CAD build for the part. Positions are in the model's coordinates, mm. A direction names the side the tool comes from. Coordinates: 2 decimals unless noted, no trailing zeros. Write each loop counter-clockwise with the first axis right and the second up, starting at its lowest first coordinate (ties: lowest second). Pieces come first, ordered by that corner, then holes. Notation, with made-up numbers: (24.25, 74) -> (49.25, 74) arc R22 ccw to (49.25, 82) -> close; hole circle Ø9 at (53, 12). An arc over 180 degrees is marked (long way). Answer as CSV lines item,"result". Start each with the question number.
```python
from build123d import *

# Parameters (mm, degrees)
F1_DEPTH  = 25
F2_DEPTH  = 5
F3_R      = 5
F5_DEPTH  = 5
F6_W      = 25
F6_H      = 37.5846914337
F10_R     = 1.55
F11_DEPTH = 10
F14_DEPTH = 1
F15_DEPTH = 1
F16_DEPTH = 5
F17_DEPTH = 5


# Not quite as in the source:
# - a feature names something its author has since deleted; it is built from what else it names


with BuildPart() as f1:
    # F0 (on Right) → F1 (new body)
    with BuildSketch(Plane.YZ):
        Polygon((-1.9545168432, 38.6489601963), (-33.5964987424, 14.1788767986), (-28.2257758369, -25.4589250511), (-8.406874912, -22.7735635983), (-0.7535947717, -79.2574312341), (4.2011304595, -78.5860908709), (0.1149024355, -48.4283077234), (-0.6409071668, -42.8501701471), (-3.9713255886, -18.2705245759), (3.1545996335, -0.8816359607), (10.2805248557, 16.5072526545), (30.8972257421, 32.4510197574), (34.3548171712, 35.1249215027), (58.4291094867, 53.742590351), (55.370349062, 57.6978380884), (10.2805248557, 22.8279692467), align=None)
        Polygon((-25.8654488138, -5.6400241263), (-7.3142972833, -13.2422419285), (-9.1963342424, -17.8348428934), (-23.9423909688, -19.8328594567), align=None, mode=Mode.SUBTRACT)
        Polygon((1.5615552233, 8.4168698067), (-1.4719884671, 1.0143288458), (-4.5055321574, -6.3882121151), (-5.26391808, -8.2388473554), (-11.7411414209, -5.5844966263), (-17.2930471416, -3.3093388585), (-23.7702704824, -0.6549881294), (-23.0118845598, 1.1956471108), (-16.944797179, 16.0007290327), (-16.1864112564, 17.851364273), (-9.7091879156, 15.1970135439), (-4.1572821949, 12.9218557761), (2.3199411459, 10.267505047), align=None, mode=Mode.SUBTRACT)
        Polygon((-14.6534166938, 22.50764705), (-2.8510041559, 31.6349520341), (6.2523573083, 19.863500585), (4.1741345282, 14.7921613112), align=None, mode=Mode.SUBTRACT)
        Polygon((-10.4675738382, 13.3463783036), (-4.9156681175, 11.0712205358), (-4.1572821949, 12.9218557761), (-9.7091879156, 15.1970135439), align=None)
        Polygon((-11.7411414209, -5.5844966263), (-10.9827554983, -3.7338613861), (-16.534661219, -1.4587036183), (-17.2930471416, -3.3093388585), align=None)
        Polygon((43.3848339814, 23.4483111776), (34.3548171712, 35.1249215027), (30.8972257421, 32.4510197574), (37.9390681356, 23.3452947817), (11.4856577492, -41.2070815569), (-0.6409071668, -42.8501701471), (0.1149024355, -48.4283077234), (14.7421520123, -46.4463889317), align=None)
    extrude(amount=F1_DEPTH)

    # F0 (on Right) → F2 (join)
    with BuildSketch(Plane.YZ):
        Polygon((-16.944797179, 16.0007290327), (-10.4675738382, 13.3463783036), (-9.7091879156, 15.1970135439), (-16.1864112564, 17.851364273), align=None)
        Polygon((-4.9156681175, 11.0712205358), (1.5615552233, 8.4168698067), (2.3199411459, 10.267505047), (-4.1572821949, 12.9218557761), align=None)
        Polygon((-17.2930471416, -3.3093388585), (-16.534661219, -1.4587036183), (-23.0118845598, 1.1956471108), (-23.7702704824, -0.6549881294), align=None)
        Polygon((-5.26391808, -8.2388473554), (-4.5055321574, -6.3882121151), (-10.9827554983, -3.7338613861), (-11.7411414209, -5.5844966263), align=None)
    extrude(amount=F2_DEPTH)

    # F3
    f3_edges = [f1.edges().sort_by_distance(p)[0] for p in [
        (12.5, -33.596499, 14.178877),
    ]]
    fillet(f3_edges, radius=F3_R)

    # F4 (on face) → F5 (cut)
    with BuildSketch(Plane(origin=(0, 28.9192447, -11.8510377387), x_dir=(-1, 0, 0), z_dir=(0, 0.9253176201, -0.3791929613))):
        Polygon((-25, 33.3185826418), (-25, -32.5577652662), (-18.2082508509, 0.3804086878), align=None)
        Polygon((-14.2606471901, -5.2335595779), (-20, -32.3875417919), (-4.8253758508, -32.3875417919), align=None)
        Polygon((-11.0385, 0.3804086878), (0, -31.3875417919), (0, 32.1483591675), align=None)
        with BuildLine():
            ThreePointArc((-13.1233754255, 0.3804086878), (-14.6233754255, 1.8804086878), (-16.1233754255, 0.3804086878))
            Line((-16.1233754255, 0.3804086878), (-13.1233754255, 0.3804086878))
        make_face()
        with BuildLine():
            Line((-13.1233754255, 0.3804086878), (-16.1233754255, 0.3804086878))
            ThreePointArc((-16.1233754255, 0.3804086878), (-14.6233754255, -1.1195913122), (-13.1233754255, 0.3804086878))
        make_face()
        Polygon((-5, 33.1483591675), (-20, 33.1483591675), (-14.3256804669, 6.3097710203), align=None)
    extrude(amount=-F5_DEPTH, mode=Mode.SUBTRACT)

    # F8 (on offset) → F9 section 0
    with BuildSketch(Plane(origin=(0, 12.2635275379, -5.0255644353), x_dir=(-1, 0, 0), z_dir=(0, 0.9253176201, -0.3791929613))):
        with BuildLine():
            ThreePointArc((-17.1248646707, 2.8558931882), (-18.1499909365, 0.381019454), (-17.1248646707, -2.0938542801))
            ThreePointArc((-17.1248646707, -2.0938542801), (-14.6499909365, -3.118980546), (-12.1751172024, -2.0938542801))
            ThreePointArc((-12.1751172024, -2.0938542801), (-11.1499909365, 0.381019454), (-12.1751172024, 2.8558931882))
            ThreePointArc((-12.1751172024, 2.8558931882), (-14.6499909365, 3.881019454), (-17.1248646707, 2.8558931882))
        make_face()
    # F6 (on face) → F9 section 1
    with BuildSketch(Plane(origin=(0, 3.0103513367, -1.2336348224), x_dir=(-1, 0, 0), z_dir=(0, 0.9253176201, -0.3791929613))):
        with Locations((-12.5, 0.3804086878)):
            Rectangle(F6_W, F6_H)
    loft()

    # F10 (on face) → F11 (cut)
    with BuildSketch(Plane(origin=(0, 12.2635275379, -5.0255644353), x_dir=(-1, 0, 0), z_dir=(0, 0.9253176201, -0.3791929613))):
        with Locations((-14.6499909461, 0.3810196067)):
            Circle(F10_R)
    extrude(amount=-F11_DEPTH, mode=Mode.SUBTRACT)

    # F13 (on face) → F14 (join)
    with BuildSketch(Plane(origin=(0, -11.2853910764, -1.5291137632), x_dir=(1, 0, 0), z_dir=(0, -0.9909450462, -0.1342680726))):
        with BuildLine():
            ThreePointArc((14, -43.6885751417), (16, -45.6885751417), (18, -43.6885751417))
            ThreePointArc((18, -43.6885751417), (16, -41.6885751417), (14, -43.6885751417))
        make_face()
        with BuildLine():
            Line((18, -56.1885751417), (18, -43.6885751417))
            ThreePointArc((18, -43.6885751417), (16, -45.6885751417), (14, -43.6885751417))
            Line((14, -43.6885751417), (14, -56.1885751417))
            ThreePointArc((14, -56.1885751417), (16, -54.1885751417), (18, -56.1885751417))
        make_face()
        with BuildLine():
            ThreePointArc((14, -56.1885751417), (16, -58.1885751417), (18, -56.1885751417))
            ThreePointArc((18, -56.1885751417), (16, -54.1885751417), (14, -56.1885751417))
        make_face()
    extrude(amount=F14_DEPTH)

    # F12 (on face) → F15 (join)
    with BuildSketch(Plane(origin=(0, -7.1996627103, 9.3098006026), x_dir=(1, 0, 0), z_dir=(0, -0.6117520849, 0.7910495475))):
        with BuildLine():
            ThreePointArc((14, 56.8474623166), (16, 54.8474623166), (18, 56.8474623166))
            ThreePointArc((18, 56.8474623166), (16, 58.8474623166), (14, 56.8474623166))
        make_face()
        with BuildLine():
            Line((18, 44.3474623166), (18, 56.8474623166))
            ThreePointArc((18, 56.8474623166), (16, 54.8474623166), (14, 56.8474623166))
            Line((14, 56.8474623166), (14, 44.3474623166))
            ThreePointArc((14, 44.3474623166), (16, 46.3474623166), (18, 44.3474623166))
        make_face()
        with BuildLine():
            ThreePointArc((14, 44.3474623166), (16, 42.3474623166), (18, 44.3474623166))
            ThreePointArc((18, 44.3474623166), (16, 46.3474623166), (14, 44.3474623166))
        make_face()
    extrude(amount=F15_DEPTH)

    # F12 (on face) → F16 (cut)
    with BuildSketch(Plane(origin=(0, -7.1996627103, 9.3098006026), x_dir=(1, 0, 0), z_dir=(0, -0.6117520849, 0.7910495475))):
        with BuildLine():
            ThreePointArc((14, 64.8474623166), (16, 62.8474623166), (18, 64.8474623166))
            ThreePointArc((18, 64.8474623166), (16, 66.8474623166), (14, 64.8474623166))
        make_face()
        with BuildLine():
            ThreePointArc((14, 36.3474623166), (16, 34.3474623166), (18, 36.3474623166))
            ThreePointArc((18, 36.3474623166), (16, 38.3474623166), (14, 36.3474623166))
        make_face()
    extrude(amount=-F16_DEPTH, mode=Mode.SUBTRACT)

    # F13 (on face) → F17 (cut)
    with BuildSketch(Plane(origin=(0, -11.2853910764, -1.5291137632), x_dir=(1, 0, 0), z_dir=(0, -0.9909450462, -0.1342680726))):
        with BuildLine():
            ThreePointArc((14, -35.6885751417), (16, -37.6885751417), (18, -35.6885751417))
            ThreePointArc((18, -35.6885751417), (16, -33.6885751417), (14, -35.6885751417))
        make_face()
        with BuildLine():
            ThreePointArc((14, -64.1885751417), (16, -66.1885751417), (18, -64.1885751417))
            ThreePointArc((18, -64.1885751417), (16, -62.1885751417), (14, -64.1885751417))
        make_face()
    extrude(amount=-F17_DEPTH, mode=Mode.SUBTRACT)


solid = f1.part
```
1. Wall check: line 1 (Y direction, x = 13, z = 24); line 2 (Y direction, x = 12.5, z = -14.5); line 3 (Z direction, x = 8.5, y = 0). Give the ranges that are in metal, low to high.
2. Cut at C-C (z = 40). Give the cut face in (x, y).
3. Cut at A-A (z = -27.5). Give the cut face in (x, y).
4. Tool access for faces 4 (the face through (12.32, 7.33, -47.45)), 5 (the face through (5, -13, 16)), 6 (the face through (12.325, -5.108, 18.596)), 7 (the face through (14.672, 3.163, -0.861)), 8 (the face through (15.972, 32.305, 41.125)): list every direction of +Z, -Z, +X, -X, +Y, -Y with a clear straight run to the whole face (end or side of a thin tool).
5. Flat gauge pins, fed straight in: P1, Ø1, axis at x = 22, z = 41, coming from the +Y side; P2, Ø4, axis at x = 22, y = 35.5, coming from the -Z side; P3, Ø1.4, axis at y = -2.5, z = 11, coming from the +X side. Where does each tip first touch, or does it go through?
6. Mould opens along X. For faces 1 (the face through (12.32, 1.64, 25.83)), 2 (the face through (14, -5, -51)), 3 (the face through (14, -4.1, -36.5)) say: pulls with the +X half, pulls with the -X half, needs draft (parallel to the pull), parting line crosses it, or undercut.
7. Cut at B-B (x = 8.75). Count the separate pieces of the cut face and the enclosed holes in it, then the cut area to 3 significant figures.
Geometry check:
1,line 1,"-20.9 to -12.72, 3.05 to 9.37, 11.8 to 19.97, 37.43 to 42.96"
1,line 2,"-29.71 to -24.66, -7.83 to 1.5, 22.43 to 27.83"
1,line 3,"-79.16 to -42.76, -15.5 to 4.61, 11.22 to 16.5, 27.95 to 36.12"
2,outline,"(0, 32.49) -> (14, 32.49) -> (14, 30.85) -> (18, 30.85) -> (18, 32.49) -> (25, 32.49) -> (25, 40.66) -> (0, 40.66) -> close"
3,outline,"(0, -7.77) -> (25, -7.77) -> (25, -2.72) -> (0, -2.72) -> close; (4.32, 17.1) -> (9.49, 17.1) -> (10.2, 22.51) -> (5.03, 22.51) -> close; (16.73, 22.51) -> (17.16, 17.1) -> (22.2, 17.1) -> (21.77, 22.51) -> close"
4,face 4,"+X, -X, +Y"
4,face 5,"+X"
4,face 6,"+X, -X"
4,face 7,"none"
4,face 8,"+Z, +X, -X"
5,P1,"y = 42.6"
5,P2,"z = 0.25"
5,P3,"x = 5"
6,face 1,"needs draft"
6,face 2,"pulls with the -X half"
6,face 3,"undercut"
7,separate pieces,"3"
7,enclosed holes,"3"
7,area,"2,230 mm²"
